```python
from build123d import *

# Parameters (mm, degrees)
SKETCH1_R           = 1.5
BOSS_EXTRUDE1_DEPTH = 2
SKETCH2_R           = 3.5
SKETCH2_R_2         = 1.5
BOSS_EXTRUDE2_DEPTH = 7
SKETCH3_R           = 3.5
SKETCH3_R_2         = 1.5
BOSS_EXTRUDE3_DEPTH = 15
SKETCH4_R           = 3.5
SKETCH4_R_2         = 1.5
BOSS_EXTRUDE4_DEPTH = 2


with BuildPart() as part:
    # Sketch1 → Boss-Extrude1 (new body)
    with BuildSketch(Plane.XY):
        with BuildLine():
            Line((-35, 43.5), (80, 43.5))
            ThreePointArc((80, 43.5), (83.5, 40), (80, 36.5))
            Line((80, 36.5), (6.5, 36.5))
            ThreePointArc((6.5, 36.5), (4.378679656, 35.621320344), (3.5, 33.5))
            Line((3.5, 33.5), (3.5, 0))
            ThreePointArc((3.5, 0), (0, -3.5), (-3.5, 0))
            Line((-3.5, 0), (-3.5, 33.5))
            ThreePointArc((-3.5, 33.5), (-4.378679656, 35.621320344), (-6.5, 36.5))
            Line((-6.5, 36.5), (-35, 36.5))
            ThreePointArc((-35, 36.5), (-38.5, 40), (-35, 43.5))
        make_face()
        with Locations((-35, 40)):
            Circle(SKETCH1_R, mode=Mode.SUBTRACT)
        with Locations((80, 40)):
            Circle(SKETCH1_R, mode=Mode.SUBTRACT)
        Circle(SKETCH1_R, mode=Mode.SUBTRACT)
    extrude(amount=BOSS_EXTRUDE1_DEPTH)

    # Sketch2 → Boss-Extrude2 (add)
    with BuildSketch(Plane.XY.offset(2)):
        with Locations(Location((-35, 40, 0), (0, 0, 270))):
            Circle(SKETCH2_R)
        with Locations((-35, 40)):
            Circle(SKETCH2_R_2, mode=Mode.SUBTRACT)
    extrude(amount=BOSS_EXTRUDE2_DEPTH)

    # Sketch3 → Boss-Extrude3 (add)
    with BuildSketch(Plane.XY.offset(2)):
        with Locations(Location((80, 40, 0), (0, 0, 90))):
            Circle(SKETCH3_R)
        with Locations((80, 40)):
            Circle(SKETCH3_R_2, mode=Mode.SUBTRACT)
    extrude(amount=BOSS_EXTRUDE3_DEPTH)

    # Sketch4 → Boss-Extrude4 (add)
    with BuildSketch(Plane.XY.offset(2)):
        Circle(SKETCH4_R)
        Circle(SKETCH4_R_2, mode=Mode.SUBTRACT)
    extrude(amount=BOSS_EXTRUDE4_DEPTH)


solid = part.part
```
The model under review builds one solid part; all positions refer to its coordinate system, in mm. A direction names the side the tool comes from. Round coordinates to 2 decimals unless told otherwise and drop trailing zeros. Loops run counter-clockwise (first coordinate to the right, second up) from the corner with the lowest first, then second, coordinate; pieces in that order, holes last.
Item 1: For faces 1 (the face through (83.417, 39.241, 8.381)), 2 (the face through (3.5, 17, 1)), 3 (the face through (-21, 36.5, 1)), list the 3-axis set-ups (+Z, -Z, +X, -X, +Y, -Y) from which the entire face can be reached by the end or side of a thin tool; tool diameter is ignored.
Determined:
face 1: +Z
face 2: +Z, -Z, +X, -Y
face 3: +Z, -Z, -X, -Y
Item 2: Take a section at B-B (y = 40). Write out the cut boundary in (x, z), then the cut area to 3 significant figures.
Determined:
outline: (-38.5, 0) - (-36.5, 0) - (-36.5, 9) - (-38.5, 9) - close; (-33.5, 0) - (78.5, 0) - (78.5, 17) - (76.5, 17) - (76.5, 2) - (-31.5, 2) - (-31.5, 9) - (-33.5, 9) - close; (81.5, 0) - (83.5, 0) - (83.5, 17) - (81.5, 17) - close
area: 320 mm2
Item 3: For line 1 (Y direction, x = 80, z = 8.5); line 2 (Y direction, x = 0, z = 1.55); line 3 (X direction, y = 31.5, z = 1), list the stretches that pass through material, from the lowest coordinate up.
Determined:
line 1: y = 36.5 to 38.5, 41.5 to 43.5
line 2: y = -3.5 to -1.5, 1.5 to 43.5
line 3: x = -3.5 to 3.5
Item 4: Clearance check with flat-ended pins moving along their axes: pin 1 Ø4 at (x, y) = (3, 35.5) entering from -Z; pin 2 Ø5.5 at (x, y) = (-36, 40.5) entering from +Z; pin 3 Ø2 at (x, y) = (-1, -1) entering from +Z; pin 4 Ø0.6 at (x, z) = (55.5, 1) entering from -Y. State where each tip first meets the part, or that it passes through.
Determined:
pin 1: stops at z = 0
pin 2: stops at z = 9
pin 3: stops at z = 4
pin 4: stops at y = 36.5
Item 5: Take a section at C-C (z = 13.75). Write out the cut boundary in (x, y), then the cut area to 3 significant figures.
Determined:
outline: circle Ø7 at (80, 40); hole circle Ø3 at (80, 40)
area: 31.4 mm2
Item 6: Take a section at D-D (y = 14). Write out the cut boundary in (x, z).
Determined:
outline: (-3.5, 0) - (3.5, 0) - (3.5, 2) - (-3.5, 2) - close
Item 7: Mouldability with a two-part tool opening along X and no side actions: class faces 4 (the face through (0, -2, 4)), 5 (the face through (4.4, 35.64, 0.99)), 6 (the face through (-36.2, 39.1, 4.4)) as released by +X, released by -X, zero draft, split by the parting line, or undercut.
Determined:
face 4: zero draft
face 5: released by +X
face 6: undercut
Item 8: Take a section at A-A (x = 0). Write out the cut boundary in (y, z), then the cut area to 3 significant figures.
Determined:
outline: (-3.5, 0) - (-1.5, 0) - (-1.5, 4) - (-3.5, 4) - close; (1.5, 0) - (43.5, 0) - (43.5, 2) - (3.5, 2) - (3.5, 4) - (1.5, 4) - close
area: 96.0 mm2
